from build123d import *

# Parameters (mm, degrees)
SKETCH1_W                 = 155
SKETCH1_H                 = 180
BOSS_EXTRUDE1_DEPTH       = 4
FILLET1_R                 = 5
F_4_0MM_DOWEL_HOLE1_D     = 4
F_4_0MM_DOWEL_HOLE1_DEPTH = 3.1
SKETCH4_R                 = 1.95
CUT_EXTRUDE1_DEPTH        = 238.573146631
SKETCH5_R                 = 2.8
CUT_EXTRUDE2_DEPTH        = 3.1
CUT_EXTRUDE3_START        = -1.5
CUT_EXTRUDE3_DEPTH        = 1.5


with BuildPart() as part:
    # Sketch1 → Boss-Extrude1 (new body)
    with BuildSketch(Plane.XY):
        with Locations((77.5, 90)):
            Rectangle(SKETCH1_W, SKETCH1_H)
    extrude(amount=BOSS_EXTRUDE1_DEPTH)

    # Fillet1
    fillet1_edges = [part.edges().sort_by_distance(p)[0] for p in [
        (0, 180, 2),
        (155, 180, 2),
        (155, 0, 2),
        (0, 0, 2),
    ]]
    fillet(fillet1_edges, radius=FILLET1_R)

    # Ø4.0mm Dowel Hole1
    with Locations(Plane(origin=(0, 0, 0), x_dir=(-1, 0, 0), z_dir=(0, 0, -1))):
        with Locations((-60.95, 31.55), (-60.95, 61.55), (-61.95, 77.25), (-53.55, 107.55), (-61.95, 159.35), (-28.85, 107.55), (-22.6, 37.42), (-100.2, 19.55), (-98.45, 47.3), (-98.45, 75.05), (-110.45, 149.65), (-70.45, 149.65), (-70.45, 100.725), (-94.08, 100.725), (-148.75, 98.75), (-148.75, 127.85), (-148.75, 165.75), (-148.75, 136.65), (-141, 54.55), (-141, 34.05), (-137.55, 73.15), (-35.35, 50.590757681), (-125.355437925, 9.944755633), (-141, 9.944755633), (-141, 25.620981812), (-125.355437925, 25.620981812)):
            Hole(F_4_0MM_DOWEL_HOLE1_D / 2, depth=F_4_0MM_DOWEL_HOLE1_DEPTH)

    # Sketch4 → Cut-Extrude1 (cut, through all)
    with BuildSketch(Plane(origin=(0, 0, 0), x_dir=(-1, 0, 0), z_dir=(0, 0, -1))):
        with Locations((-5.5, 5.5)):
            Circle(SKETCH4_R)
        with Locations((-5.5, 90)):
            Circle(SKETCH4_R)
        with Locations((-5.5, 174.5)):
            Circle(SKETCH4_R)
        with Locations(Location((-149.5, 174.5, 0), (0, 0, 180))):
            Circle(SKETCH4_R)
        with Locations(Location((-149.5, 90, 0), (0, 0, 180))):
            Circle(SKETCH4_R)
        with Locations(Location((-149.5, 5.5, 0), (0, 0, 180))):
            Circle(SKETCH4_R)
    extrude(amount=-CUT_EXTRUDE1_DEPTH, mode=Mode.SUBTRACT)

    # Sketch5 → Cut-Extrude2 (cut)
    with BuildSketch(Plane.XY.offset(4)):
        with Locations((149.5, 5.5)):
            Circle(SKETCH5_R)
        with Locations((149.5, 90)):
            Circle(SKETCH5_R)
        with Locations((149.5, 174.5)):
            Circle(SKETCH5_R)
        with Locations((5.5, 174.5)):
            Circle(SKETCH5_R)
        with Locations((5.5, 90)):
            Circle(SKETCH5_R)
        with Locations((5.5, 5.5)):
            Circle(SKETCH5_R)
    extrude(amount=-CUT_EXTRUDE2_DEPTH, mode=Mode.SUBTRACT)

    # Sketch6 → Cut-Extrude3 (cut)
    with BuildSketch(Plane(origin=(0, 0, 0), x_dir=(-1, 0, 0), z_dir=(0, 0, -1)).offset(CUT_EXTRUDE3_START)):
        with BuildLine():
            Line((-150, 0), (-5, 0))
            ThreePointArc((-5, 0), (-1.464466094, 1.464466094), (0, 5))
            Line((0, 5), (0, 175))
            ThreePointArc((0, 175), (-1.464466094, 178.535533906), (-5, 180))
            Line((-5, 180), (-150, 180))
            ThreePointArc((-150, 180), (-153.535533906, 178.535533906), (-155, 175))
            Line((-155, 175), (-155, 5))
            ThreePointArc((-155, 5), (-153.535533906, 1.464466094), (-150, 0))
        make_face()
        with BuildLine():
            Line((-150, 1.2), (-5, 1.2))
            ThreePointArc((-5, 1.2), (-2.312994231, 2.312994231), (-1.2, 5))
            Line((-1.2, 5), (-1.2, 175))
            ThreePointArc((-1.2, 175), (-2.312994231, 177.687005769), (-5, 178.8))
            Line((-5, 178.8), (-150, 178.8))
            ThreePointArc((-150, 178.8), (-152.687005769, 177.687005769), (-153.8, 175))
            Line((-153.8, 175), (-153.8, 5))
            ThreePointArc((-153.8, 5), (-152.687005769, 2.312994231), (-150, 1.2))
        make_face(mode=Mode.SUBTRACT)
    extrude(amount=CUT_EXTRUDE3_DEPTH, mode=Mode.SUBTRACT)


solid = part.part
Can you work these out from the model? Positions are in its coordinate system, mm. A direction names the side the tool comes from. Give positions to 0.01 mm unless a question says otherwise; leave off trailing zeros. Write each loop counter-clockwise with the first axis right and the second up, starting at its lowest first coordinate (ties: lowest second). Pieces come first, ordered by that corner, then holes. Notation, with made-up numbers: (-5.5, 17) -> (53.5, 17) arc R26 cw to (53.5, 34) -> close; hole circle Ø3 at (82.5, -32). An arc over 180 degrees is marked (long way). Answer as a JSON object with one key per item and string values. Group by question number.
Item 1: Suppose I cut it at A-A (x = 22.6). Please give me the cut outline in (y, z), plus the area to 3 significant figures.
Item 2: Please list where these lines run through material, in increasing order: line 1 (X direction, y = 149.65, z = 1.4); line 2 (Y direction, x = 5.5, z = 2.45); line 3 (Y direction, x = 59.5, z = 0.3). Write a range as [from, to].
Item 3: For faces 1 (the face through (150.548, 172.856, 0.444)), 2 (the face through (62, 159, 3.1)), 3 (the face through (7.3, 88.8, 0.9)), which set-ups out of +Z, -Z, +X, -X, +Y, -Y let a thin tool reach every point of the face, with its end or its side?
Item 4: Suppose I cut it at B-B (y = 19.55). Please give me the cut outline in (x, z), plus the area to 3 significant figures.
Item 5: I'm going to push flat-ended pins straight in: P1, Ø6, axis at x = 20, y = 56.5, coming from the -Z side; P2, Ø3, axis at x = 5, y = 175.5, coming from the +Z side; P3, Ø1.2, axis at x = 99.5, y = 47, coming from the -Z side. Where does each tip first touch, or does it pass through?
Findings:
{
 "1": {"outline": "(0, 1.5) -> (1.2, 1.5) -> (1.2, 0) -> (35.42, 0) -> (35.42, 3.1) -> (39.42, 3.1) -> (39.42, 0) -> (178.8, 0) -> (178.8, 1.5) -> (180, 1.5) -> (180, 4) -> (0, 4) -> close", "area": "704 mm²"},
 "2": {"line 1": "x = [1.2, 68.45], [72.45, 108.45], [112.45, 153.8]", "line 2": "y = [0, 2.7], [8.3, 87.2], [92.8, 171.7], [177.3, 180]", "line 3": "y = [1.2, 30.17], [32.93, 60.17], [62.93, 178.8]"},
 "3": {"face 1": "+Z, -Z", "face 2": "-Z", "face 3": "+Z"},
 "4": {"outline": "(0, 1.5) -> (1.2, 1.5) -> (1.2, 0) -> (98.2, 0) -> (98.2, 3.1) -> (102.2, 3.1) -> (102.2, 0) -> (153.8, 0) -> (153.8, 1.5) -> (155, 1.5) -> (155, 4) -> (0, 4) -> close", "area": "604 mm²"},
 "5": {"P1": "stops at z = 0", "P2": "stops at z = 0.9", "P3": "stops at z = 3.1"}
}
